Verification items for the finished model (mm, model axes). Face numbers are marked on the shaded views. A direction names the side the tool comes from. Coordinates: 2 decimals unless noted, no trailing zeros. Write each loop counter-clockwise with the first axis right and the second up, starting at its lowest first coordinate (ties: lowest second). Pieces come first, ordered by that corner, then holes. Notation, with made-up numbers: M 86.25,-17 L 119.25,-17 A23 ccw 119.25,21 Z; hole C 7,-5.75 d10. An arc over 180 degrees is marked long. One line per item, written item: value.
```python
from build123d import *

# Parameters (mm, degrees)
BOSS_EXTRUDE1_DEPTH = 5.35


with BuildPart() as part:
    # Model → Boss-Extrude1 (new body)
    with BuildSketch(Plane.XY):
        with BuildLine():
            Line((-29, 0), (29, 0))
            Line((29, 0), (29, -5.35))
            Line((29, -5.35), (35, -5.35))
            Line((35, -5.35), (35, -1.30660388))
            Line((35, -1.30660388), (35, 7.65))
            Line((35, 7.65), (30, 7.65))
            Line((30, 7.65), (30, 13))
            Line((30, 13), (35, 13))
            Line((35, 13), (35, 26))
            Line((35, 26), (28.495613698, 26))
            ThreePointArc((28.495613698, 26), (28.145175376, 25.856641252), (27.99569065, 25.50877193))
            ThreePointArc((27.99569065, 25.50877193), (27.297393866, 19.766839637), (25.434173666, 14.290909091))
            ThreePointArc((25.434173666, 14.290909091), (25.249671939, 14.078962321), (24.979991994, 14))
            Line((24.979991994, 14), (24.213890642, 14))
            ThreePointArc((24.213890642, 14), (23.953774224, 13.927012236), (23.76959907, 13.729357798))
            ThreePointArc((23.76959907, 13.729357798), (22.402719166, 11.382179575), (20.804862314, 9.185714286))
            ThreePointArc((20.804862314, 9.185714286), (20.631459285, 9.048811094), (20.415986383, 9))
            Line((20.415986383, 9), (17.224924528, 9))
            ThreePointArc((17.224924528, 9), (17.035413911, 8.962693987), (16.874182835, 8.856342904))
            ThreePointArc((16.874182835, 8.856342904), (0, 1.945), (-16.874182835, 8.856342904))
            ThreePointArc((-16.874182835, 8.856342904), (-17.035413911, 8.962693987), (-17.224924528, 9))
            Line((-17.224924528, 9), (-20.415986383, 9))
            ThreePointArc((-20.415986383, 9), (-20.631459285, 9.048811094), (-20.804862314, 9.185714286))
            ThreePointArc((-20.804862314, 9.185714286), (-22.402719166, 11.382179575), (-23.76959907, 13.729357798))
            ThreePointArc((-23.76959907, 13.729357798), (-23.953774224, 13.927012236), (-24.213890642, 14))
            Line((-24.213890642, 14), (-24.979991994, 14))
            ThreePointArc((-24.979991994, 14), (-25.249671939, 14.078962321), (-25.434173666, 14.290909091))
            ThreePointArc((-25.434173666, 14.290909091), (-27.297393866, 19.766839637), (-27.99569065, 25.50877193))
            ThreePointArc((-27.99569065, 25.50877193), (-28.145175376, 25.856641252), (-28.495613698, 26))
            Line((-28.495613698, 26), (-35, 26))
            Line((-35, 26), (-35, 13))
            Line((-35, 13), (-30, 13))
            Line((-30, 13), (-30, 7.65))
            Line((-30, 7.65), (-35, 7.65))
            Line((-35, 7.65), (-35, -1.30660388))
            Line((-35, -1.30660388), (-35, -5.35))
            Line((-35, -5.35), (-29, -5.35))
            Line((-29, -5.35), (-29, 0))
        make_face()
    extrude(amount=BOSS_EXTRUDE1_DEPTH)


solid = part.part
```
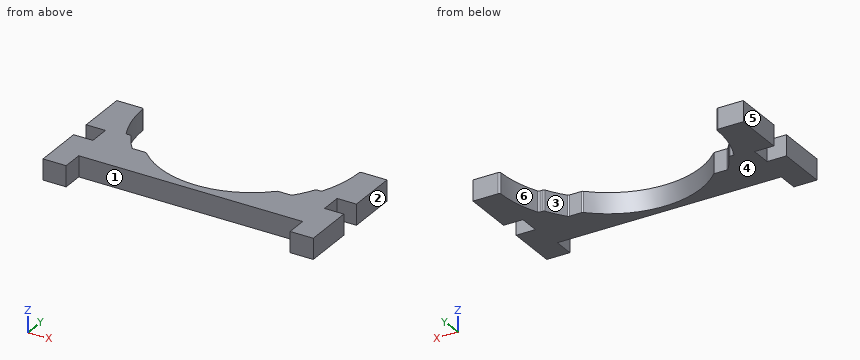
Item 1: Cross-section at D-D, the plane x = -7. Enter the section's corners in (y, z), and give its area (3 significant figures).
The answers:
outline: M 0,0 L 2.99,0 L 2.99,5.35 L 0,5.35 Z
area: 16.0 mm²
Item 2: Go/stop test with flat-tipped pins: P1, Ø1, axis at x = -18, z = 4, coming from the +Y side; P2, Ø1.5, axis at x = 23.5, z = 1, coming from the +Y side; P3, Ø1, axis at x = -11, z = 5, coming from the -Y side. Record where each tip stops, or that it passes through.
The answers:
P1: stops at y = 9
P2: stops at y = 14
P3: stops at y = 0
Item 3: Access from +Z, -Z, +X, -X, +Y, -Y to the whole of each face (thin tool, end or side, straight path). Record for the marked faces 1, 2 and 3.
The answers:
face 1: +Z, -Z, -Y
face 2: +Z, -Z, +X, +Y, -Y
face 3: +Z, -Z, +Y
Item 4: Cross-section at B-B, the plane y = 20.5. Enter the section's corners in (x, z).
The answers:
outline: M -35,0 L -27.45,0 L -27.45,5.35 L -35,5.35 Z; M 27.45,0 L 35,0 L 35,5.35 L 27.45,5.35 Z
Item 5: Scan lines: line 1 (Y direction, x = 31, z = 4.05); line 2 (X direction, y = -4, z = 1.9); line 3 (X direction, y = 12, z = 4.7). Record each from-to range of solid material in increasing order.
The answers:
line 1: y = -5.35 to 7.65, 13 to 26
line 2: x = -35 to -29, 29 to 35
line 3: x = -30 to -22.79, 22.79 to 30
Item 6: Draft check along X on the marked faces 4, 5 and 6. Enter one of: released by +X, released by -X, zero draft, split by the parting line, or undercut.
The answers:
face 4: zero draft
face 5: released by -X
face 6: undercut
Item 7: Cross-section at A-A, the plane y = -2.5. Enter the section's corners in (x, z).
The answers:
outline: M -35,0 L -29,0 L -29,5.35 L -35,5.35 Z; M 29,0 L 35,0 L 35,5.35 L 29,5.35 Z
Item 8: Cross-section at C-C, the plane x = -19. Enter the section's corners in (y, z), and give its area (4 significant figures).
The answers:
outline: M 0,0 L 9,0 L 9,5.35 L 0,5.35 Z
area: 48.15 mm²
